The listing builds one solid part. Answer for the finished solid, in the listing's coordinates (mm). Face numbers are marked on the shaded views. Round coordinates to 2 decimals unless told otherwise and drop trailing zeros. Write each loop counter-clockwise with the first axis right and the second up, starting at its lowest first coordinate (ties: lowest second). Pieces come first, ordered by that corner, then holes.
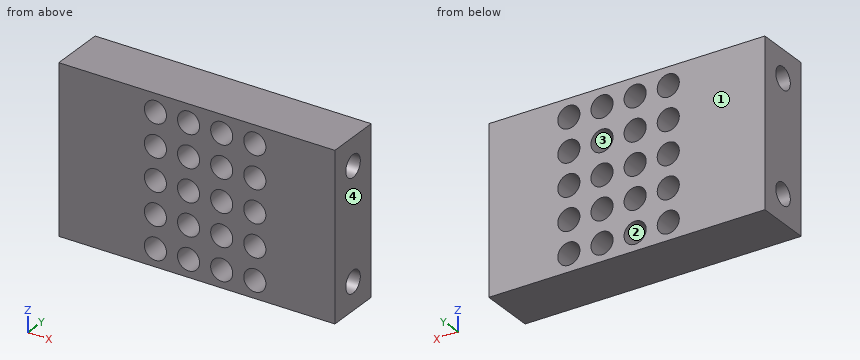
Autodesk Inventor part; units mm, degrees
ref_plane "YZ Plane" through (0, 0, 0) normal (1, 0, 0) x (0, 1, 0)
ref_plane "XZ Plane" through (0, 0, 0) normal (0, 1, 0) x (-1, 0, 0)
ref_plane "XY Plane" through (0, 0, 0) normal (0, 0, 1) x (1, 0, 0)
sketch "Sketch1" plane through (0, 0, 0) normal (0, 1, 0) x (-1, 0, 0)
  line L0 (-4.0944, 5.5957) -> (45.9056, 5.5957)
  line L1 (45.9056, 5.5957) -> (45.9056, -24.4043)
  line L2 (45.9056, -24.4043) -> (-4.0944, -24.4043)
  line L3 (-4.0944, -24.4043) -> (-4.0944, 5.5957)
  point P0 (0, 0)
  dimension "d0" = 50
  dimension "d1" = 30
extrude "Extrusion1" add sketch "Sketch1" along normal blind 10
sketch "Sketch2" plane through (4.0944, 0, 5.5957) normal (1, 0, 0) x (0, 0, -1)
  line L0 (30, 0) -> (0, 0)
  line L1 (15, 0) -> (15, 10)
  line L2 (30, 10) -> (0, 10)
  line L3 (15, 5) -> (5, 5)
  line L4 (15, 5) -> (25, 5)
  circle A0 centre (5, 5) radius 2
  circle A1 centre (25, 5) radius 2
  point P0 (5.5957, 0)
  dimension "d4" = 10
  dimension "d5" = 10
  dimension "d6" = 4
  dimension "d7" = 4
extrude "Extrusion2" cut sketch "Sketch2" against normal blind 10
sketch "Sketch3" plane through (-45.9056, 0, -24.4043) normal (-1, 0, 0) x (0, 0, 1)
  line L0 (30, 0) -> (0, 0)
  line L1 (15, 0) -> (15, 10)
  line L2 (30, 10) -> (0, 10)
  line L3 (15, 5) -> (5, 5)
  line L4 (15, 5) -> (25, 5)
  circle A0 centre (5, 5) radius 2
  circle A1 centre (5, 5) radius 2
  circle A2 centre (25, 5) radius 2
  circle A3 centre (25, 5) radius 2
  point P0 (24.4043, 0)
  dimension "d10" = 10
  dimension "d11" = 10
extrude "Extrusion3" cut sketch "Sketch3" against normal blind 10
sketch "Sketch4" plane through (0, 10, 0) normal (0, 1, 0) x (1, 0, 0)
  line L0 (-45.9056, 24.4043) -> (-45.9056, -5.5957)
  line L1 (-45.9056, 9.4043) -> (4.0944, 9.4043)
  line L2 (4.0944, -5.5957) -> (4.0944, 24.4043)
  line L3 (-20.9056, 9.4043) -> (-20.9056, -5.5957)
  line L4 (-45.9056, -5.5957) -> (4.0944, -5.5957)
  line L5 (-20.9056, 9.4043) -> (-20.9056, 24.4043)
  line L6 (-20.9056, 16.9043) -> (-35.9056, 16.9043)
  line L7 (-45.9056, 17.4043) -> (-35.9056, 17.4043)
  line L8 (-20.9056, 16.9043) -> (-5.9056, 16.9043)
  line L9 (-5.9056, 1.4043) -> (-5.9056, -2.5957)
  line L10 (-20.9056, 1.4043) -> (-5.9056, 1.4043)
  line L11 (-20.9056, 1.4043) -> (-35.9056, 1.4043)
  line L12 (-28.4056, 16.9043) -> (-28.4056, -5.5957)
  line L13 (-28.4056, 24.4043) -> (-28.4056, -5.5957)
  line L14 (-28.4056, 16.9043) -> (-20.9056, 16.9043)
  line L15 (-20.9056, 9.4043) -> (-28.4056, 9.4043)
  line L16 (-20.9056, 1.4043) -> (-28.4056, 1.4043)
  line L17 (-20.9056, 0) -> (-28.4056, 0)
  circle A0 centre (-28.4056, 21.2599) radius 2
  circle A1 centre (-28.4056, 21.2599) radius 2
  circle A2 centre (-28.4056, 15.3599) radius 2
  circle A3 centre (-28.4056, 9.4599) radius 2
  circle A4 centre (-28.4056, 3.5599) radius 2
  circle A5 centre (-28.4056, -2.3401) radius 2
  circle A6 centre (-22.4056, 21.2599) radius 2
  circle A7 centre (-22.4056, 15.3599) radius 2
  circle A8 centre (-22.4056, 9.4599) radius 2
  circle A9 centre (-22.4056, 3.5599) radius 2
  circle A10 centre (-22.4056, -2.3401) radius 2
  circle A11 centre (-16.4056, 21.2599) radius 2
  circle A12 centre (-16.4056, 15.3599) radius 2
  circle A13 centre (-16.4056, 9.4599) radius 2
  circle A14 centre (-16.4056, 3.5599) radius 2
  circle A15 centre (-16.4056, -2.3401) radius 2
  circle A16 centre (-10.4056, 21.2599) radius 2
  circle A17 centre (-10.4056, 15.3599) radius 2
  circle A18 centre (-10.4056, 9.4599) radius 2
  circle A19 centre (-10.4056, 3.5599) radius 2
  circle A20 centre (-10.4056, -2.3401) radius 2
  point P0 (0, 0)
  dimension "d17" = 4
  dimension "d27" = 5.9
  dimension "d30" = 6
extrude "Extrusion4" cut sketch "Sketch4" against normal blind 10 contours A0 L13 | L13 A0 | A6 L5 | L5 A6 | A17 L8 | L8 A17 | A12 L8 | L8 A12 | A3 L12 L1 | L1 L12 A3 | L12 A3 L1 | L1 A3 L12 | A5 L12 | L12 A5 | A2 L6 L12 | L12 L6 A2 | A4 L12 | L12 A4 | A10 L3 | L3 A10 | A8 L5 L1 | L1 L3 A8 | L13 A2 L6 | L6 A2 L13 | L5 A8 L1 | L1 A8 L3 | A18 L1 | L1 A18 | A7 L6 L5 | L5 A7 | A9 L3 | L3 A9 | A7 L6 | A13 L1 | L1 A13 | A11 | A14 | A15 | A16 | A19 | A20 picked at (-21.946, 15.7701)
thread "Thread1"
thread "Thread2"
thread "Thread3"
thread "Thread4"
properties part number "cubito pro max"
1. Section D-D on y = 8 is taken. Give the number of separate pieces and of enclosed holes in the cut face, plus the area to 3 significant figures.
Geometry says:
separate pieces: 1
enclosed holes: 20
area: 1,250 mm2
2. Section C-C on z = -8 is taken. Determine the outline of the cut face in (x, y), plus the area to 3 significant figures.
Geometry says:
outline: (-45.91, 0) - (-29.77, 0) - (-29.77, 10) - (-45.91, 10) - close; (-27.04, 0) - (-23.77, 0) - (-23.77, 10) - (-27.04, 10) - close; (-21.04, 0) - (-17.77, 0) - (-17.77, 10) - (-21.04, 10) - close; (-15.04, 0) - (-11.77, 0) - (-11.77, 10) - (-15.04, 10) - close; (-9.04, 0) - (4.09, 0) - (4.09, 10) - (-9.04, 10) - close
area: 391 mm2
3. Given pin 1 (3 mm diameter, centred on y = 5, z = 0.6, fed in from +X); pin 2 (2.5 mm diameter, centred on y = 5, z = -19.4, fed in from -X), each flat-ended and moving along its own axis, determine where each tip first touches the part or whether it passes through.
Geometry says:
pin 1: stops at x = -5.91
pin 2: stops at x = -35.91
4. Section B-B on x = -41 is taken. Determine the outline of the cut face in (y, z), plus the area to 3 significant figures.
Geometry says:
outline: (0, -24.4) - (10, -24.4) - (10, 5.6) - (0, 5.6) - close; hole circle Ø4 at (5, -19.4); hole circle Ø4 at (5, 0.6)
area: 275 mm2
5. Section A-A on x = -11 is taken. Determine the outline of the cut face in (y, z).
Geometry says:
outline: (0, -24.4) - (10, -24.4) - (10, -23.17) - (0, -23.17) - close; (0, -19.35) - (10, -19.35) - (10, -17.27) - (0, -17.27) - close; (0, -13.45) - (10, -13.45) - (10, -11.37) - (0, -11.37) - close; (0, -7.55) - (10, -7.55) - (10, -5.47) - (0, -5.47) - close; (0, -1.65) - (10, -1.65) - (10, 0.43) - (0, 0.43) - close; (0, 4.25) - (10, 4.25) - (10, 5.6) - (0, 5.6) - close
6. For a pull along X with two mould halves and no side action, classify the marked faces 1, 2, 3 and 4 as released by +X, released by -X, zero draft, split by the parting line, or undercut.
Geometry says:
face 1: zero draft
face 2: undercut
face 3: undercut
face 4: released by +X
7. Straight lines are drawn through the part: line 1 along Z through (x, y) = (-15.5, 8); line 2 along Z through (x, y) = (-37, 6); line 3 along X through (y, z) = (5, 1.75). For each, find the intervals that lie inside material, in ascending order.
Geometry says:
line 1: z = -24.4 to -23.04, -19.48 to -17.14, -13.58 to -11.24, -7.68 to -5.34, -1.78 to 0.56, 4.12 to 5.6
line 2: z = -24.4 to -21.14, -17.67 to -1.14, 2.33 to 5.6
line 3: x = -35.91 to -30.32, -26.49 to -24.32, -20.49 to -18.32, -14.49 to -12.32, -8.49 to -5.91
